Could you check a few things on this drawing? It's one solid part, dimensions in mm from its lowest x, y, z. A direction names the side the tool comes from. Give positions to 0.01 mm unless a question says otherwise; leave off trailing zeros. Loops run counter-clockwise (first coordinate to the right, second up) from the corner with the lowest first, then second, coordinate; pieces in that order, holes last. Notation, with made-up numbers: (64, 85.5) - (93, 85.5) arc R19 ccw to (93, 98.5) - close; hole circle Ø1 at (57.5, -36). An arc over 180 degrees is marked (long way). Write each question's results on one line, items separated by ' | '. Start each with the question number.
(1) I need wall thicknesses on line 1 (X direction, y = 21.5, z = 0.7); line 2 (Y direction, x = 4.5, z = 3.4); line 3 (X direction, y = 8.5, z = 1.85). Which ranges of each line are inside material? Lowest first, please.
(2) On a 3-axis mill with a long thin cutter (end or side, diameter ignored), from which of +Z, -Z, +X, -X, +Y, -Y can I reach the whole of each face in a straight line? I mean the marked faces 4, 5 and 6. Say none if no direction works.
(3) Suppose I cut it at C-C (y = 15.5). Please give me the cut outline in (x, z), and give its area (3 significant figures).
(4) Suppose I cut it at D-D (x = 34). Please give me the cut outline in (y, z), and give its area (3 significant figures).
(5) Suppose I cut it at B-B (x = 6). Please give me the cut outline in (y, z).
(6) Suppose I cut it at A-A (x = 40.5). Please give me the cut outline in (y, z).
(7) For pin 1 (1.5 mm diameter, centred on y = 17, z = 2, fed in from -X); pin 2 (2 mm diameter, centred on x = 21.5, z = 2, fed in from +Y); pin 3 (0.7 mm diameter, centred on y = 21, z = 2, fed in from +X), each with a flat end and sliding along its axis, tell me the tip position at first contact or that it passes through.
(8) If we mould it in two halves opening along Y, with no side actions, what happens to the marked faces 1, 2 and 3? For each: released by +Y, released by -Y, zero draft, split by the parting line, or undercut.
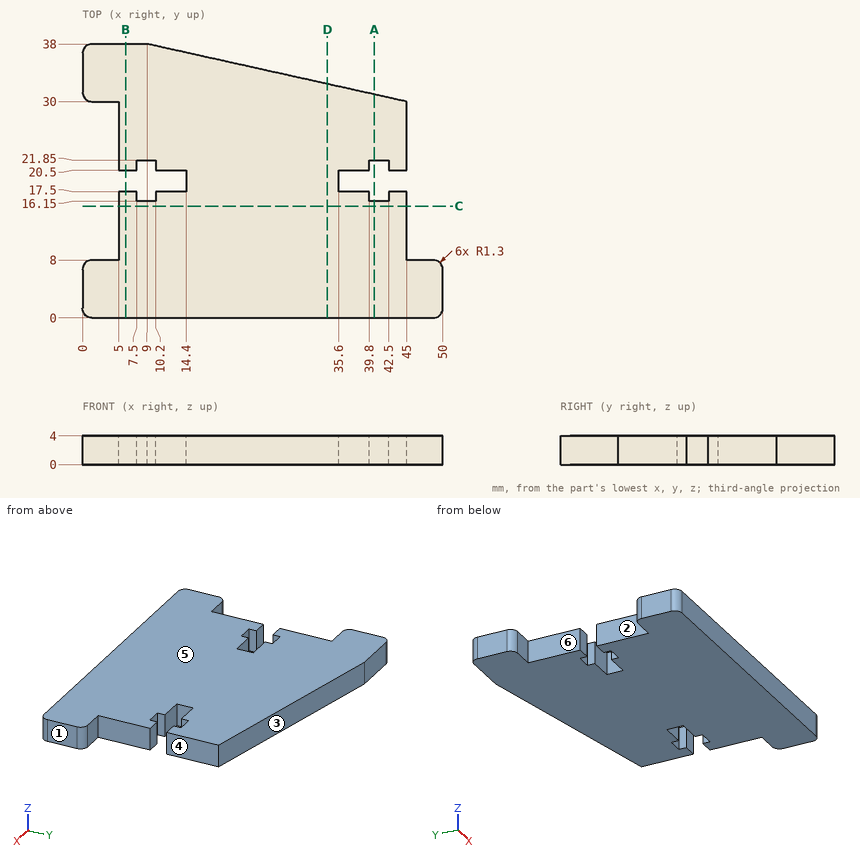
Output values:
1) line 1: 5 to 7.5, 10.2 to 39.8, 42.5 to 45 | line 2: 0 to 8, 30 to 38 | line 3: 5 to 45
2) face 4: +Z, -Z, +X, +Y | face 5: +Z, +X, -X, +Y, -Y | face 6: +Z, -Z, -X
3) outline: (5, 0) - (45, 0) - (45, 4) - (5, 4) - close | area: 160 mm2
4) outline: (0, 0) - (32.44, 0) - (32.44, 4) - (0, 4) - close | area: 130 mm2
5) outline: (0, 0) - (17.5, 0) - (17.5, 4) - (0, 4) - close; (20.5, 0) - (38, 0) - (38, 4) - (20.5, 4) - close
6) outline: (0, 0) - (16.15, 0) - (16.15, 4) - (0, 4) - close; (21.85, 0) - (31, 0) - (31, 4) - (21.85, 4) - close
7) pin 1: x = 5 | pin 2: y = 35.44 | pin 3: x = 45
8) face 1: zero draft | face 2: undercut | face 3: released by +Y
